Autodesk Inventor part; units mm, degrees
ref_plane "YZ Plane" through (0, 0, 0) normal (1, 0, 0) x (0, 1, 0)
ref_plane "XZ Plane" through (0, 0, 0) normal (0, 1, 0) x (-1, 0, 0)
ref_plane "XY Plane" through (0, 0, 0) normal (0, 0, 1) x (1, 0, 0)
sketch "Sketch1" plane through (0, 0, 0) normal (0, 1, 0) x (-1, 0, 0)
  circle A0 centre (0, 0) radius 45
  circle A1 centre (0, 0) radius 35
  line L0 (35, 0) -> (45, 0)
  line L1 (45, 0) -> (45, 40)
  line L2 (45, 40) -> (35, 40)
  line L3 (35, 40) -> (35, 0)
  line L4 (-0.1589, -34.9996) -> (-40.1589, -34.9996)
  line L5 (-40.1589, -34.9996) -> (-40.1589, -44.9997)
  line L6 (-40.1589, -44.9997) -> (-0.1589, -44.9997)
  line L7 (-0.1589, -44.9997) -> (-0.1589, -34.9996)
  point P0 (-0.1589, -44.9997)
  point P1 (45, 0)
  point P2 (-28.2847, -34.9996)
  point P3 (35, 28.2843)
  point P4 (-0.1589, -44.9997)
  dimension "d0" = 90
  dimension "d1" = 70
  dimension "d2" = 40
  dimension "d3" = 40
extrude "Extrusion1" add sketch "Sketch1" along normal blind 10 contours L7 A1 L0 A0 | L6 L5 L4 A0 | A0 L4 L7 | L0 L3 A0 | A0 L3 L2 L1
chamfer "Chamfer1" distance 9 angle 45 3 edges at (-35, 0, 20) (-24.6925, 0, -24.8048) (20.1589, 0, -34.9996)
equation "\"BendRadius\" = Thickness"
equation "\"BendReliefWidth\" = Thickness"
equation "\"BendReliefDepth\" = 0.5 * Thickness"
equation "\"CornerReliefSize\" = 4 * Thickness"
equation "\"MinimumRemnant\" = 2 * Thickness"
equation "\"TransitionRadius\" = BendRadius"
equation "\"JacobiRadiusSize\" = BendRadius"
equation "\"GapSize\" = Thickness"
properties part number "test1"
The model under review builds one solid part; all positions refer to its coordinate system, in mm. A direction names the side the tool comes from. Round coordinates to 2 decimals unless told otherwise and drop trailing zeros. Write each loop counter-clockwise with the first axis right and the second up, starting at its lowest first coordinate (ties: lowest second). Pieces come first, ordered by that corner, then holes. Notation, with made-up numbers: (-28, 75) - (28, 75) arc R7 ccw to (28, 88) - close; hole circle Ø8 at (-14, 47.5). An arc over 180 degrees is marked (long way). Use one line per item in the form item = value.
Q1. For line 1 (X direction, y = 5.5, z = -14.5); line 2 (X direction, y = 6.25, z = 20.5); line 3 (Z direction, x = -5.5, y = 4.25), list the stretches that pass through material, from the lowest coordinate up. Write a range as [from, to].
Answer key:
line_1 = [-42.6, -35.67]
line_2 = [-45, -37.75]
line_3 = [-44.66, -39.37]
Q2. Insertion check: pin 1 Ø3 at (x, y) = (24, 6.5) entering from +Z; pin 2 Ø2 at (y, z) = (8.5, 1) entering from +X; pin 3 Ø1.1 at (x, y) = (12, 9.5) entering from +Z. Each pin has a flat end and moves straight along its axis. Give the tip position at first contact, or say it passes through.
Answer key:
pin_1 = -36
pin_2 = -35
pin_3 = -35
Q3. Consider section A-A (x = 29). State the section outline as (y, z) points, and give its area (3 significant figures).
Answer key:
outline = (0, -45) - (10, -45) - (10, -35) - (9, -35) - (0, -44) - close
area = 59.5 mm2
Q4. Consider section B-B (y = 3.75). State the section outline as (x, z) points, and give its area (3 significant figures).
Answer key:
outline = (-45, 0) arc R45 ccw to (0.16, -45) - (40.16, -45) - (40.16, -40.25) - (0.18, -40.25) arc R40.25 cw to (-40.25, 0) - (-40.25, 40) - (-45, 40) - close
area = 699 mm2
Q5. Consider section D-D (y = 8). State the section outline as (x, z) points.
Answer key:
outline = (-45, 0) arc R45 ccw to (0.16, -45) - (40.16, -45) - (40.16, -36) - (0.16, -36) arc R36 cw to (-36, 0) - (-36, 40) - (-45, 40) - close
Q6. Tool access review of faces 1 (the flat face through (-27, 10, -24)), 2 (the flat face through (-40, 4, 20)): name each direction out of +Z, -Z, +X, -X, +Y, -Y from which nothing blocks a thin tool from reaching the whole face with its end or side.
Answer key:
face_1 = +Z, -Z, +X, -X, +Y
face_2 = +Z, +X, -Y
Q7. Consider section C-C (z = 20.5). State the section outline as (x, y) points, and give its area (3 significant figures).
Answer key:
outline = (-45, 0) - (-44, 0) - (-35, 9) - (-35, 10) - (-45, 10) - close
area = 59.5 mm2
